Source: CAD feature listing. Evaluate the final solid. Frame: model axes, mm. Face numbers are marked on the shaded views. Round coordinates to 2 decimals unless told otherwise and drop trailing zeros. Write each loop counter-clockwise with the first axis right and the second up, starting at its lowest first coordinate (ties: lowest second). Pieces come first, ordered by that corner, then holes. Notation, with made-up numbers: M 82,84.5 L 90,84.5 A20 cw 90,89.5 Z; hole C 74,-34.75 d10. An arc over 180 degrees is marked long. Answer in a Markdown table with one row per item.
from build123d import *

# Parameters (mm, degrees)
SKETCH1_W                = 5.5
SKETCH1_H                = 2.5
BOSS_EXTRUDE1_DEPTH      = 2.5
BOSS_EXTRUDE2_START      = -10.8
SKETCH2_W                = 0.6
SKETCH2_H                = 0.6
BOSS_EXTRUDE2_DEPTH      = 13.3
CHAMFER1_SIZE            = 0.2
CHAMFER1_OF_MIRROR1_SIZE = 0.2


with BuildPart() as part:
    # Sketch1 → Boss-Extrude1 (new body)
    with BuildSketch(Plane(origin=(0, 0, 0), x_dir=(1, 0, 0), z_dir=(0, 1, 0))):
        Rectangle(SKETCH1_W, SKETCH1_H)
    extrude(amount=BOSS_EXTRUDE1_DEPTH)

    # Sketch2 → Boss-Extrude2 (add)
    with BuildSketch(Plane(origin=(0, 2.5, 0), x_dir=(1, 0, 0), z_dir=(0, 1, 0)).offset(BOSS_EXTRUDE2_START)):
        with Locations((-1.25, 0)):
            Rectangle(SKETCH2_W, SKETCH2_H)
    boss_extrude2 = extrude(amount=BOSS_EXTRUDE2_DEPTH)

    # Chamfer1
    chamfer1_edges = [part.edges().sort_by_distance(p)[0] for p in [
        (-1.55, -8.3, 0),
        (-1.25, -8.3, -0.3),
        (-0.95, -8.3, 0),
        (-1.25, -8.3, 0.3),
        (-1.55, 5, 0),
        (-1.25, 5, 0.3),
        (-0.95, 5, 0),
        (-1.25, 5, -0.3),
    ]]
    chamfer(chamfer1_edges, length=CHAMFER1_SIZE)

    # Mirror1: Boss-Extrude2 across plane
    add(boss_extrude2.mirror(Plane(origin=(0, 0, 0), x_dir=(0, 0, 1), z_dir=(1, 0, 0))))

    # Chamfer1 of Mirror1
    chamfer1_of_mirror1_edges = [part.edges().sort_by_distance(p)[0] for p in [
        (1.55, -8.3, 0),
        (1.25, -8.3, -0.3),
        (0.95, -8.3, 0),
        (1.25, -8.3, 0.3),
        (1.55, 5, 0),
        (1.25, 5, 0.3),
        (0.95, 5, 0),
        (1.25, 5, -0.3),
    ]]
    chamfer(chamfer1_of_mirror1_edges, length=CHAMFER1_OF_MIRROR1_SIZE)


solid = part.part
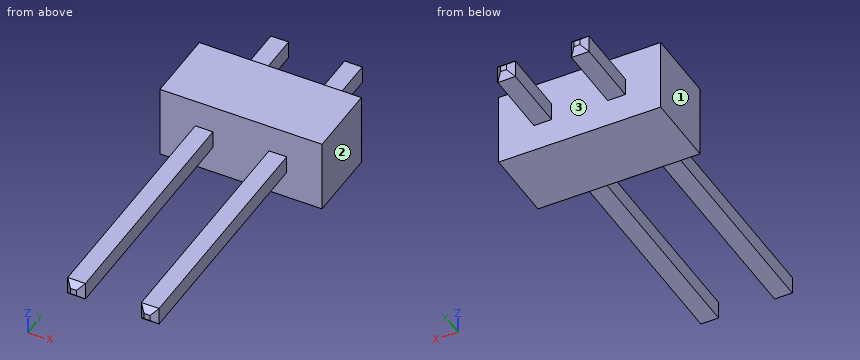
Q1. Section C-C (x = 0.1). Return loops of the section in (y, z), and give its area (3 significant figures).
Solutions:
| item | result |
|---|---|
| outline | M 0,-1.25 L 2.5,-1.25 L 2.5,1.25 L 0,1.25 Z |
| area | 6.25 mm2 |
Q2. Pull-direction query (X, two-part tool) for the marked faces 1, 2 and 3; classes: pulls with the +X half, pulls with the -X half, needs draft (parallel to the pull), parting line crosses it, or undercut.
Solutions:
| item | result |
|---|---|
| face 1 | pulls with the -X half |
| face 2 | pulls with the +X half |
| face 3 | undercut |
Q3. Section B-B (z = -1). Return loops of the section in (x, y), and give its area (4 significant figures).
Solutions:
| item | result |
|---|---|
| outline | M -2.75,0 L 2.75,0 L 2.75,2.5 L -2.75,2.5 Z |
| area | 13.75 mm2 |
Q4. Material intervals for probe 1 along Y at (x, z) = (2.45, -0.5); probe 2 along X at (y, z) = (-6, -0.2); probe 3 along Z at (x, y) = (-1, -3), sorted ascending.
Solutions:
| item | result |
|---|---|
| probe 1 | y = 0 to 2.5 |
| probe 2 | x = -1.55 to -0.95, 0.95 to 1.55 |
| probe 3 | z = -0.3 to 0.3 |
Q5. Contact query for flat-ended pins moving along their axis: pin 1 Ø0.7 at (y, z) = (4, 0) entering from -X; pin 2 Ø1.5 at (x, y) = (-1.5, -5) entering from -Z; pin 3 Ø0.7 at (y, z) = (-2.5, 0) entering from +X. Output: stop coordinate, or through.
Solutions:
| item | result |
|---|---|
| pin 1 | stops at x = -1.55 |
| pin 2 | stops at z = -0.3 |
| pin 3 | stops at x = 1.55 |
Q6. Section A-A (y = -0.25). Return loops of the section in (x, z), and give its area (3 significant figures).
Solutions:
| item | result |
|---|---|
| outline | M -1.55,-0.3 L -0.95,-0.3 L -0.95,0.3 L -1.55,0.3 Z; M 0.95,-0.3 L 1.55,-0.3 L 1.55,0.3 L 0.95,0.3 Z |
| area | 0.720 mm2 |
